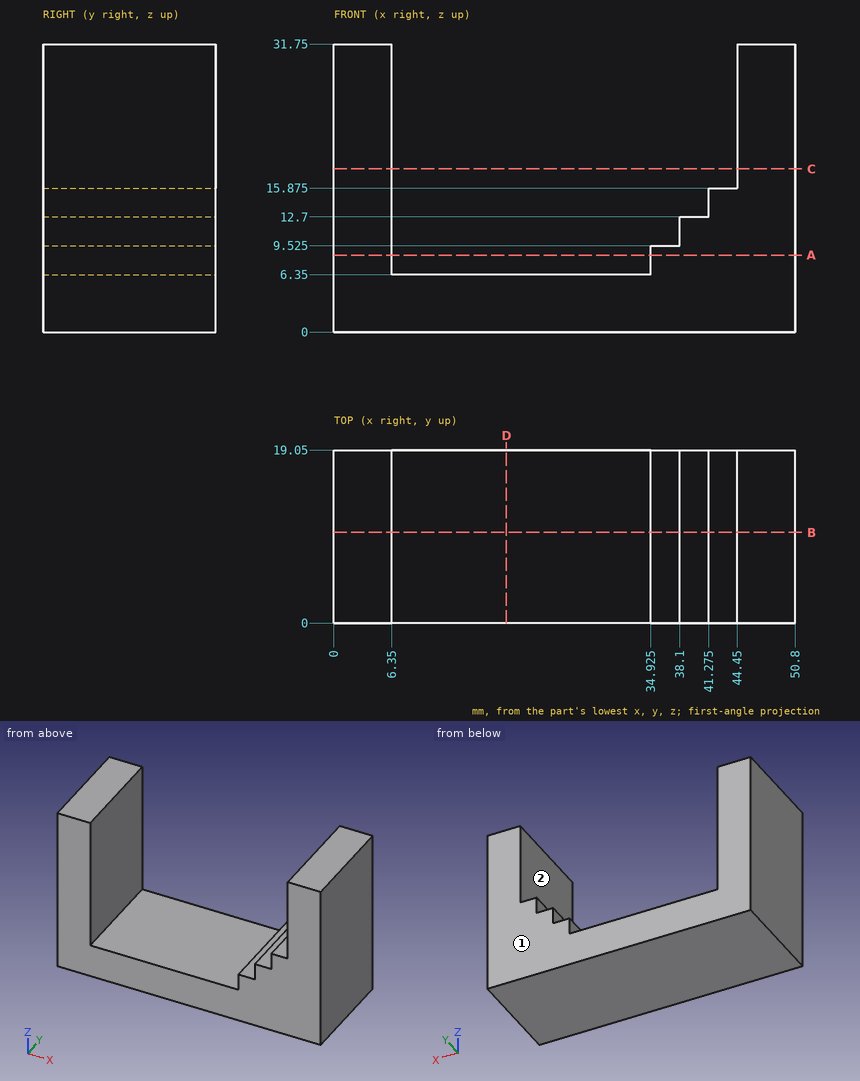
Check sheet for the drawn part. Datum: minimum x, y, z corner. Units: mm. A direction names the side the tool comes from. Round coordinates to 2 decimals unless told otherwise and drop trailing zeros. Loops run counter-clockwise (first coordinate to the right, second up) from the corner with the lowest first, then second, coordinate; pieces in that order, holes last. Notation, with made-up numbers: (81.25, 81.25) - (89.25, 81.25) arc R26 ccw to (89.25, 106.25) - close; hole circle Ø7 at (19.5, 51.25). An arc over 180 degrees is marked (long way). Write item = value, one per line. Start each with the question number.
1. Section check B-B on y = 10. Enter the section's corners in (x, z) (3 decimals).
2. Thickness scan on line 1 (X direction, y = 17, z = 28); line 2 (Z direction, x = 29, y = 6); line 3 (Z direction, x = 42, y = 11.75) (3 decimals). Record the ranges inside material, lowest first.
3. Depth check by flat-ended pin: pin 1 (8 mm diameter, centred on x = 23.5, y = 15, fed in from +Z); pin 2 (3.5 mm diameter, centred on x = 36.5, y = 11.5, fed in from +Z). Enter the tip coordinate at first touch or a pass-through.
4. Set-up check for the marked faces 1 and 2: record each of +Z, -Z, +X, -X, +Y, -Y from which the full face is reachable in a straight line by a thin tool's end or side.
5. Section check A-A on z = 8.5. Enter the section's corners in (x, y) (3 decimals).
6. Section check C-C on z = 18. Enter the section's corners in (x, y), then the cut area to 3 significant figures.
7. Section check D-D on x = 19. Enter the section's corners in (y, z), then the cut area to 3 significant figures.
Working result:
q1.outline = (0, 0) - (50.8, 0) - (50.8, 31.75) - (44.45, 31.75) - (44.45, 15.875) - (41.275, 15.875) - (41.275, 12.7) - (38.1, 12.7) - (38.1, 9.525) - (34.925, 9.525) - (34.925, 6.35) - (6.35, 6.35) - (6.35, 31.75) - (0, 31.75) - close
q2.line_1 = 0 to 6.35, 44.45 to 50.8
q2.line_2 = 0 to 6.35
q2.line_3 = 0 to 15.875
q3.pin_1 = 6.35
q3.pin_2 = 12.7
q4.face_1 = +Z, -Z, +X, -X, +Y
q4.face_2 = +Z, +Y, -Y
q5.outline = (0, 0) - (6.35, 0) - (6.35, 19.05) - (0, 19.05) - close; (34.925, 0) - (50.8, 0) - (50.8, 19.05) - (34.925, 19.05) - close
q6.outline = (0, 0) - (6.35, 0) - (6.35, 19.05) - (0, 19.05) - close; (44.45, 0) - (50.8, 0) - (50.8, 19.05) - (44.45, 19.05) - close
q6.area = 242 mm^2
q7.outline = (0, 0) - (19.05, 0) - (19.05, 6.35) - (0, 6.35) - close
q7.area = 121 mm^2
